from build123d import *

# Parameters (mm, degrees)
FILLET1_R = 0.5


with BuildPart() as part:
    # Sweep1: sweep along a path in Sketch2path
    with BuildLine(Plane.XY) as sweep1_path:
        Line((0, 100), (10, 100))
        ThreePointArc((10, 100), (80.430596643, 89.552607894), (144.795757594, 59.110153969))
        Line((144.795757594, 59.110153969), (153.110453717, 53.554451639))
    # Sketch3 → Sweep1 (sweep)
    with BuildSketch(Plane(origin=(0, 0, 0), x_dir=(0, 0, -1), z_dir=(1, 0, 0))):
        with BuildLine():
            Line((-5, 106), (5, 106))
            ThreePointArc((5, 106), (11, 100), (5, 94))
            Line((5, 94), (-5, 94))
            ThreePointArc((-5, 94), (-11, 100), (-5, 106))
        make_face()
        with BuildLine():
            Line((-5, 105), (5, 105))
            ThreePointArc((5, 105), (10, 100), (5, 95))
            Line((5, 95), (-5, 95))
            ThreePointArc((-5, 95), (-10, 100), (-5, 105))
        make_face(mode=Mode.SUBTRACT)
    sweep(path=sweep1_path.line)

    # Fillet1
    fillet1_edges = [part.edges().sort_by_distance(p)[0] for p in [
        (0, 100, -10),
        (0, 105, 0),
        (0, 100, 10),
        (153.110453717, 53.554451639, 10),
        (150.332602552, 49.397103578, 0),
        (153.110453717, 53.554451639, -10),
        (155.888304882, 57.711799701, 0),
        (0, 95, 0),
    ]]
    fillet(fillet1_edges, radius=FILLET1_R)


solid = part.part
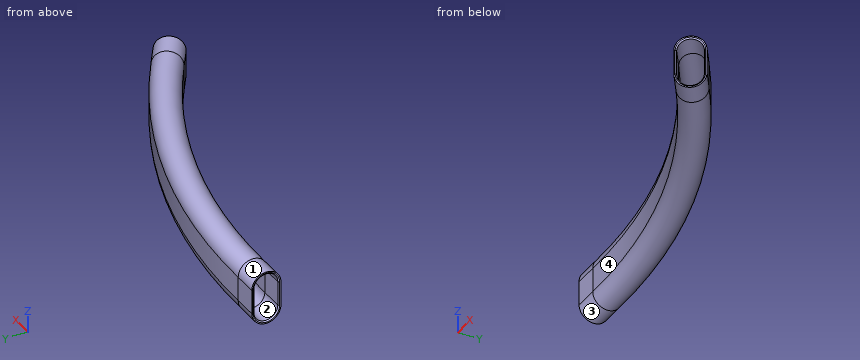
Part model, mm, in its own coordinate system. Face numbers are marked on the shaded views. Coordinates: 2 decimals unless noted, no trailing zeros. Order: outer loops, then holes, each group sorted by start corner. A loop starts at its lowest first (then second) coordinate and runs counter-clockwise, first axis right, second up.
(1) Probe L1, parallel to Z at x = 144.5, y = 59.5; L2, parallel to Z at x = 60, y = 91.5; L3, parallel to X at y = 73, z = 0. List the from-to ranges inside material, lowest first.
Check sheet entries:
L1: z = -11 to -10, 10 to 11
L2: z = -10.06 to -8.82, 8.82 to 10.06
L3: x = 107.45 to 109.86, 131.75 to 133.78
(2) Pull direction Z, two halves, no side cores. Call the marked faces 1, 2, 3 and 4: pulls with the +Z half, pulls with the -Z half, needs draft (parallel to the pull), parting line crosses it, or undercut.
Check sheet entries:
face 1: pulls with the +Z half
face 2: undercut
face 3: pulls with the -Z half
face 4: needs draft
(3) Slice it at A-A, the plane z = -1. Write the cut outline in (x, y).
Check sheet entries:
outline: (0, 94) - (10, 94) arc R236.63 cw to (141.46, 54.12) - (149.78, 48.57) - (150.05, 48.98) arc R0.5 ccw to (149.92, 49.67) - (142.02, 54.95) arc R237.63 ccw to (10, 95) - (0.5, 95) arc R0.5 ccw to (0, 94.5) - close; (0, 105.5) arc R0.5 ccw to (0.5, 105) - (10, 105) arc R247.63 cw to (147.57, 63.27) - (155.47, 57.99) arc R0.5 ccw to (156.17, 58.13) - (156.44, 58.54) - (148.13, 64.1) arc R248.63 ccw to (10, 106) - (0, 106) - close
(4) Pin check, flat tips, straight feed: pin 1 Ø4 at (x, z) = (122.5, 5) entering from +Y (3 decimals); pin 2 Ø3 at (x, z) = (43, -7) entering from +Y; pin 3 Ø5 at (x, z) = (85, 7) entering from -Y. Stop position of each tip, or through.
Check sheet entries:
pin 1: stops at y = 80.095
pin 2: stops at y = 103.87
pin 3: stops at y = 81.11
